```python
from build123d import *

# Parameters (mm, degrees)
SKETCH1_W           = 60
SKETCH1_H           = 80
BOSS_EXTRUDE1_DEPTH = 5
SKETCH2_R           = 2
CUT_EXTRUDE1_DEPTH  = 5
SKETCH3_W           = 7
SKETCH3_H           = 2
CUT_EXTRUDE2_DEPTH  = 5
FILLET2_R           = 10


with BuildPart() as part:
    # Sketch1 → Boss-Extrude1 (new body)
    with BuildSketch(Plane.XY):
        with Locations((-30, 40)):
            Rectangle(SKETCH1_W, SKETCH1_H)
    extrude(amount=BOSS_EXTRUDE1_DEPTH)

    # Sketch2 → Cut-Extrude1 (cut)
    with BuildSketch(Plane.XY.offset(5)):
        with Locations((-51, 40)):
            Circle(SKETCH2_R)
        with Locations((-9, 64.411542732)):
            Circle(SKETCH2_R)
        with Locations((-9, 15.588457268)):
            Circle(SKETCH2_R)
    extrude(amount=-CUT_EXTRUDE1_DEPTH, mode=Mode.SUBTRACT)

    # Sketch3 → Cut-Extrude2 (cut)
    with BuildSketch(Plane.XY.offset(5)):
        with Locations((-51, 69)):
            Rectangle(SKETCH3_W, SKETCH3_H)
        with Locations((-51, 62)):
            Rectangle(SKETCH3_W, SKETCH3_H)
        with Locations((-51, 18)):
            Rectangle(SKETCH3_W, SKETCH3_H)
        with Locations((-51, 11)):
            Rectangle(SKETCH3_W, SKETCH3_H)
    extrude(amount=-CUT_EXTRUDE2_DEPTH, mode=Mode.SUBTRACT)

    # Fillet2
    fillet2_edges = [part.edges().sort_by_distance(p)[0] for p in [
        (-60, 0, 2.5),
        (-60, 80, 2.5),
        (0, 80, 2.5),
        (0, 0, 2.5),
    ]]
    fillet(fillet2_edges, radius=FILLET2_R)


solid = part.part
```
Work out the finished part from the listing and answer in its coordinate system (mm). A direction names the side the tool comes from. Give positions to 0.01 mm unless a question says otherwise; leave off trailing zeros. Write each loop counter-clockwise with the first axis right and the second up, starting at its lowest first coordinate (ties: lowest second). Pieces come first, ordered by that corner, then holes.
(1) The part is cut by section A-A on y = 40. Write down the section's boundary in (x, z).
Final values:
outline: (-60, 0) - (-53, 0) - (-53, 5) - (-60, 5) - close; (-49, 0) - (0, 0) - (0, 5) - (-49, 5) - close
(2) The mould has two halves that part along Y. Classify faces 1 (the flat face through (-30, 0, 2)), 2 (the flat face through (-30, 80, 2)), 3 (the flat face through (-51, 19, 3)): pulls with the +Y half, pulls with the -Y half, needs draft (parallel to the pull), parting line crosses it, or undercut.
Final values:
face 1: pulls with the -Y half
face 2: pulls with the +Y half
face 3: undercut
(3) The part is cut by section D-D on y = 69. Write down the section's boundary in (x, z), plus the area to 3 significant figures.
Final values:
outline: (-60, 0) - (-54.5, 0) - (-54.5, 5) - (-60, 5) - close; (-47.5, 0) - (0, 0) - (0, 5) - (-47.5, 5) - close
area: 265 mm2
(4) The part is cut by section C-C on z = 1.05. Write down the section's boundary in (x, y), plus the area to 3 significant figures.
Final values:
outline: (-60, 10) arc R10 ccw to (-50, 0) - (-10, 0) arc R10 ccw to (0, 10) - (0, 70) arc R10 ccw to (-10, 80) - (-50, 80) arc R10 ccw to (-60, 70) - close; hole (-54.5, 10) - (-47.5, 10) - (-47.5, 12) - (-54.5, 12) - close; hole (-54.5, 17) - (-47.5, 17) - (-47.5, 19) - (-54.5, 19) - close; hole (-54.5, 61) - (-47.5, 61) - (-47.5, 63) - (-54.5, 63) - close; hole (-54.5, 68) - (-47.5, 68) - (-47.5, 70) - (-54.5, 70) - close; hole circle Ø4 at (-51, 40); hole circle Ø4 at (-9, 15.59); hole circle Ø4 at (-9, 64.41)
area: 4,620 mm2
(5) Flat-ended cylindrical pins translate along their axes: pin 1 Ø12 at (x, y) = (-7, 43.5) entering from -Z; pin 2 Ø1.5 at (x, z) = (-52, 3) entering from +Y. Find the tip coordinate at first contact, or state that the pin passes through.
Final values:
pin 1: stops at z = 0
pin 2: stops at y = 79.92
(6) The part is cut by section B-B on x = -51. Write down the section's boundary in (y, z), plus the area to 3 significant figures.
Final values:
outline: (0.05, 0) - (10, 0) - (10, 5) - (0.05, 5) - close; (12, 0) - (17, 0) - (17, 5) - (12, 5) - close; (19, 0) - (38, 0) - (38, 5) - (19, 5) - close; (42, 0) - (61, 0) - (61, 5) - (42, 5) - close; (63, 0) - (68, 0) - (68, 5) - (63, 5) - close; (70, 0) - (79.95, 0) - (79.95, 5) - (70, 5) - close
area: 339 mm2
(7) Which of the six approach directions +Z, -Z, +X, -X, +Y, -Y give full straight-line access (tool end or side, diameter ignored) to faces 4 (the flat face through (-47.5, 69, 3)), 5 (the flat face through (-30, 41, 0))?
Final values:
face 4: +Z, -Z
face 5: -Z, +X, -X, +Y, -Y
(8) Straight lines are drawn through the part: line 1 (X direction, y = 62, z = 2.55); line 2 (Y direction, x = -9, z = 3.6); line 3 (Y direction, x = -51, z = 3.8). For each, find the intervals that lie inside material, in ascending order.
Final values:
line 1: x = -60 to -54.5, -47.5 to 0
line 2: y = 0.05 to 13.59, 17.59 to 62.41, 66.41 to 79.95
line 3: y = 0.05 to 10, 12 to 17, 19 to 38, 42 to 61, 63 to 68, 70 to 79.95
